Part model, mm, in its own coordinate system. Face numbers are marked on the shaded views. A direction names the side the tool comes from. Coordinates: 2 decimals unless noted, no trailing zeros. Write each loop counter-clockwise with the first axis right and the second up, starting at its lowest first coordinate (ties: lowest second). Pieces come first, ordered by that corner, then holes. Notation, with made-up numbers: (68.5, -7) - (108.5, -7) arc R21 ccw to (108.5, 12) - close; hole circle Ø9 at (5.25, 3.25). An arc over 180 degrees is marked (long way). Use one line per item in the form item = value. Start each with the question number.
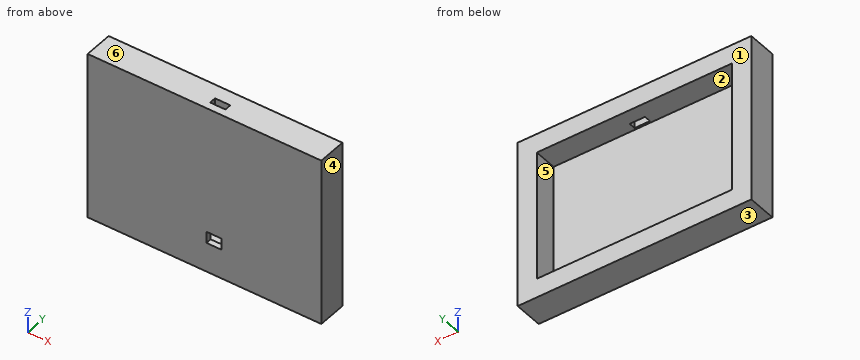
from build123d import *

# Parameters (mm, degrees)
SKETCH2_W                      = 122
SKETCH2_H                      = 88
SKETCH2_W_2                    = 102
SKETCH2_H_2                    = 68
BOSS_EXTRUDE4_DEPTH            = 15
SKETCH3_W                      = 102
SKETCH3_H                      = 68
BOSS_EXTRUDE5_DEPTH            = 3
CUT_EXTRUDE1_REACH             = 90
SKETCH4_W                      = 8
SKETCH4_H                      = 3.5
CUT_EXTRUDE1_DIRECTION_2_DEPTH = 1
SKETCH5_W                      = 8
SKETCH5_H                      = 6
CUT_EXTRUDE2_DEPTH             = 4


with BuildPart() as part:
    # Sketch2 → Boss-Extrude4 (new body)
    with BuildSketch(Plane(origin=(0, 0, 0), x_dir=(1, 0, 0), z_dir=(0, 1, 0))):
        with Locations((-31.608287026, -3.544696319)):
            Rectangle(SKETCH2_W, SKETCH2_H)
        with Locations((-31.608287026, -3.544696319)):
            Rectangle(SKETCH2_W_2, SKETCH2_H_2, mode=Mode.SUBTRACT)
    extrude(amount=BOSS_EXTRUDE4_DEPTH)

    # Sketch3 → Boss-Extrude5 (add)
    with BuildSketch(Plane(origin=(0, 0, 0), x_dir=(1, 0, 0), z_dir=(0, 1, 0))):
        with Locations((-31.608287026, -3.544696319)):
            Rectangle(SKETCH3_W, SKETCH3_H)
    extrude(amount=BOSS_EXTRUDE5_DEPTH)

    # Sketch4 → Cut-Extrude1 (cut, up to next)
    with BuildSketch(Plane.XY.offset(47.544696319), mode=Mode.PRIVATE) as cut_extrude1_sk1:
        with Locations((-27.608287026, 5.75)):
            Rectangle(SKETCH4_W, SKETCH4_H)
    cut_extrude1_tool1 = extrude(cut_extrude1_sk1.sketch, amount=-CUT_EXTRUDE1_REACH, mode=Mode.PRIVATE) & part.part
    add(cut_extrude1_tool1.solids().sort_by_distance((-27.608287, 5.75, 47.544696))[0], mode=Mode.SUBTRACT)

    # Sketch4 → Cut-Extrude1 direction 2 (cut)
    with BuildSketch(Plane.XY.offset(47.544696319)):
        with Locations((-27.608287026, 5.75)):
            Rectangle(SKETCH4_W, SKETCH4_H)
    extrude(amount=CUT_EXTRUDE1_DIRECTION_2_DEPTH, mode=Mode.SUBTRACT)

    # Sketch5 → Cut-Extrude2 (cut, through all)
    with BuildSketch(Plane(origin=(0, 3, 0), x_dir=(1, 0, 0), z_dir=(0, 1, 0))):
        with Locations((-26.608287026, 22.015303681)):
            Rectangle(SKETCH5_W, SKETCH5_H)
    extrude(amount=-CUT_EXTRUDE2_DEPTH, mode=Mode.SUBTRACT)


solid = part.part
Q1. Pin check, flat tip, straight feed: P1, Ø20.5, axis at x = -55.5, z = 14, coming from the +Y side. Stop position of the tip, or through.
Q2. Drill centre lines: probe 1 along X at (y, z) = (8.5, -13); probe 2 along Z at (x, y) = (-45.5, 12.25); probe 3 along Y at (x, z) = (-1, 13). Where is each one in solid material? Low to high.
Q3. Slice it at A-A (x = -29). List the corners of the cut face in (y, z).
Q4. Slice it at D-D (x = 17.5). List the corners of the cut face in (y, z), plus the area to 3 significant figures.
Q5. Slice it at C-C (z = -16). List the corners of the cut face in (x, y).
Q6. Which spindle directions (+Z, -Z, +X, -X, +Y, -Y) get a long thin tool onto all of the face, cutting with end or side? Do the marked faces 1 and 2. Say none if no direction does.
Q7. Mould opens along Z. For the marked faces 3, 4, 5 and 6 say: released by +Z, released by -Z, zero draft, split by the parting line, or undercut.
Q8. Slice it at B-B (y = 8.75). List the corners of the cut face in (x, z).
Solution:
q1.P1 = 3
q2.probe_1 = -92.61 to -82.61, 19.39 to 29.39
q2.probe_2 = -40.46 to -30.46, 37.54 to 47.54
q2.probe_3 = 0 to 3
q3.outline = (0, -40.46) - (15, -40.46) - (15, -30.46) - (3, -30.46) - (3, -25.02) - (0, -25.02) - close; (0, -19.02) - (3, -19.02) - (3, 37.54) - (4, 37.54) - (4, 47.54) - (0, 47.54) - close; (7.5, 37.54) - (15, 37.54) - (15, 47.54) - (7.5, 47.54) - close
q4.outline = (0, -40.46) - (15, -40.46) - (15, -30.46) - (3, -30.46) - (3, 37.54) - (15, 37.54) - (15, 47.54) - (0, 47.54) - close
q4.area = 504 mm2
q5.outline = (-92.61, 0) - (29.39, 0) - (29.39, 15) - (19.39, 15) - (19.39, 3) - (-82.61, 3) - (-82.61, 15) - (-92.61, 15) - close
q6.face_1 = +Z, -Z, +X, -X, +Y
q6.face_2 = +Y
q7.face_3 = released by -Z
q7.face_4 = zero draft
q7.face_5 = undercut
q7.face_6 = released by +Z
q8.outline = (-92.61, -40.46) - (29.39, -40.46) - (29.39, 47.54) - (-92.61, 47.54) - close; hole (-82.61, -30.46) - (19.39, -30.46) - (19.39, 37.54) - (-82.61, 37.54) - close
